Design review of the part built by this model. Coordinates are the model's own, in mm. Face numbers are marked on the shaded views. A direction names the side the tool comes from. Round coordinates to 2 decimals unless told otherwise and drop trailing zeros. Write each loop counter-clockwise with the first axis right and the second up, starting at its lowest first coordinate (ties: lowest second). Pieces come first, ordered by that corner, then holes. Notation, with made-up numbers: (-7.75, -30) -> (-2.75, -30) arc R16 cw to (-2.75, -25) -> close; hole circle Ø4 at (22, -36.5). An arc over 180 degrees is marked (long way). Write item = value, one per line. Start each with the question number.
Item 1: To check wall thickness, follow L1, parallel to Y at x = 36, z = 84; L2, parallel to X at y = 0, z = 26.5; L3, parallel to Y at x = 9, z = 46. State the ranges of each line that lie inside material, in increasing order.
Item 2: Machinability: for the marked faces 4 and 5, which of the approach directions +Z, -Z, +X, -X, +Y, -Y give a long, thin tool a straight path to every point of the face, cutting with its end or side? Answer none if there is none.
Item 3: For pin 1 Ø4 at (y, z) = (2, 61) entering from +X; pin 2 Ø6 at (x, y) = (14, 2.5) entering from +Z; pin 3 Ø6 at (y, z) = (2, 65) entering from -X, all flat-tipped, find the tip position at first contact; note any pin that passes through.
Item 4: Add section A-A, the plane x = 36. State the section outline as (y, z) points.
Item 5: Add section D-D, the plane x = 22.5. State the section outline as (y, z) points.
Item 6: Add section B-B, the plane y = 0. State the section outline as (x, z) points.
Item 7: Add section C-C, the plane z = 6. State the section outline as (x, y) points, then the cut area to 3 significant figures.
Item 8: Mouldability with a two-part tool opening along Y and no side actions: class the marked faces 1, 2 and 3 as released by +Y, released by -Y, zero draft, split by the parting line, or undercut.
from build123d import *

# Parameters (mm, degrees)
SKETCH_1_W      = 44.4
SKETCH_1_H      = 19.4
EXTRUDE_1_DEPTH = 83
FILLET_6_R      = 5
FILLET_7_R      = 5
FILLET_8_R      = 5
FILLET_9_R      = 5
FILLET_11_R     = 2
EXTRUDE_2_DEPTH = 3
EXTRUDE_START   = 3
SKETCH_3_R      = 1.2
EXTRUDE_3_DEPTH = 3


with BuildPart() as part:
    # 草图1 → 凸台-拉伸1 (new body)
    with BuildSketch(Plane.XY):
        with Locations((11.2, 0.3)):
            Rectangle(SKETCH_1_W, SKETCH_1_H)
        Polygon((-9, 6.2), (-9, -5.6), (-7.2, -5.6), (-7.2, -7.4), (29.6, -7.4), (29.6, -5.6), (31.4, -5.6), (31.4, 6.2), (29.6, 6.2), (29.6, 8), (-7.2, 8), (-7.2, 6.2), align=None, mode=Mode.SUBTRACT)
    extrude(amount=EXTRUDE_1_DEPTH)

    # 圆角6
    fillet_6_edges = [part.edges().sort_by_distance(p)[0] for p in [
        (-11, -9.4, 41.5),
    ]]
    fillet(fillet_6_edges, radius=FILLET_6_R)

    # 圆角7
    fillet_7_edges = [part.edges().sort_by_distance(p)[0] for p in [
        (-11, 10, 41.5),
    ]]
    fillet(fillet_7_edges, radius=FILLET_7_R)

    # 圆角8
    fillet_8_edges = [part.edges().sort_by_distance(p)[0] for p in [
        (33.4, 10, 41.5),
    ]]
    fillet(fillet_8_edges, radius=FILLET_8_R)

    # 圆角9
    fillet_9_edges = [part.edges().sort_by_distance(p)[0] for p in [
        (33.4, -9.4, 41.5),
    ]]
    fillet(fillet_9_edges, radius=FILLET_9_R)

    # 圆角11
    # the kernel refuses this fillet: 2 mm, written as the material it takes off along each edge
    with BuildSketch(Plane(origin=(28.4, -9.4, 0), x_dir=(0, 1, 0), z_dir=(-1, 0, 0)), Plane(origin=(-6, 10, 0), x_dir=(0, -1, 0), z_dir=(1, 0, 0))) as fillet_11_piece_1:
        with BuildLine():
            CenterArc((FILLET_11_R, -FILLET_11_R), FILLET_11_R, 90, 90)
            Line((0, -FILLET_11_R), (0, 0))
            Line((0, 0), (FILLET_11_R, 0))
        make_face()
    extrude(amount=34.4, mode=Mode.SUBTRACT)
    with BuildSketch(Plane(origin=(-6, -4.4, 0), x_dir=(0, -1, 0), z_dir=(1, 0, 0))) as fillet_11_piece_2:
        with BuildLine():
            CenterArc((5 - FILLET_11_R, -FILLET_11_R), FILLET_11_R, 0, 90)
            Line((5, -FILLET_11_R), (5, 0))
            Line((5, 0), (5 - FILLET_11_R, 0))
        make_face()
    revolve(axis=Axis((-6, -4.4, 0), (0, 0, -1)), revolution_arc=90, mode=Mode.SUBTRACT)
    with BuildSketch(Plane(origin=(-11, -4.4, 0), x_dir=(1, 0, 0), z_dir=(0, 1, 0)), Plane(origin=(33.4, 5, 0), x_dir=(-1, 0, 0), z_dir=(0, -1, 0))) as fillet_11_piece_3:
        with BuildLine():
            CenterArc((FILLET_11_R, -FILLET_11_R), FILLET_11_R, 90, 90)
            Line((0, -FILLET_11_R), (0, 0))
            Line((0, 0), (FILLET_11_R, 0))
        make_face()
    extrude(amount=9.4, mode=Mode.SUBTRACT)
    with BuildSketch(Plane(origin=(-6, 5, 0), x_dir=(-1, 0, 0), z_dir=(0, -1, 0))) as fillet_11_piece_4:
        with BuildLine():
            CenterArc((5 - FILLET_11_R, -FILLET_11_R), FILLET_11_R, 0, 90)
            Line((5, -FILLET_11_R), (5, 0))
            Line((5, 0), (5 - FILLET_11_R, 0))
        make_face()
    revolve(axis=Axis((-6, 5, 0), (0, 0, -1)), revolution_arc=90, mode=Mode.SUBTRACT)
    with BuildSketch(Plane(origin=(28.4, 5, 0), x_dir=(0, 1, 0), z_dir=(-1, 0, 0))) as fillet_11_piece_5:
        with BuildLine():
            CenterArc((5 - FILLET_11_R, -FILLET_11_R), FILLET_11_R, 0, 90)
            Line((5, -FILLET_11_R), (5, 0))
            Line((5, 0), (5 - FILLET_11_R, 0))
        make_face()
    revolve(axis=Axis((28.4, 5, 0), (0, 0, -1)), revolution_arc=90, mode=Mode.SUBTRACT)
    with BuildSketch(Plane(origin=(28.4, -4.4, 0), x_dir=(1, 0, 0), z_dir=(0, 1, 0))) as fillet_11_piece_6:
        with BuildLine():
            CenterArc((5 - FILLET_11_R, -FILLET_11_R), FILLET_11_R, 0, 90)
            Line((5, -FILLET_11_R), (5, 0))
            Line((5, 0), (5 - FILLET_11_R, 0))
        make_face()
    revolve(axis=Axis((28.4, -4.4, 0), (0, 0, -1)), revolution_arc=90, mode=Mode.SUBTRACT)

    # 草图2 → 凸台-拉伸2 (add)
    with BuildSketch(Plane(origin=(0, 0, 0), x_dir=(-1, 0, 0), z_dir=(0, 0, -1))):
        Polygon((-31.4, 6.2), (-31.4, -5.6), (-29.6, -5.6), (-29.6, -7.4), (7.2, -7.4), (7.2, -5.6), (9, -5.6), (9, 6.2), (7.2, 6.2), (7.2, 8), (-29.6, 8), (-29.6, 6.2), align=None)
    extrude(amount=-EXTRUDE_2_DEPTH)

    # 草图3 → 凸台-拉伸3 (add)
    # profile 1 of 3: a face of its own
    with BuildSketch(Plane.XY.offset(83).offset(EXTRUDE_START)):
        with BuildLine():
            Line((-6, 10), (-16, 10))
            Line((-16, 10), (-16, -9.4))
            Line((-16, -9.4), (-6, -9.4))
            ThreePointArc((-6, -9.4), (-9.535533906, -7.935533906), (-11, -4.4))
            Line((-11, -4.4), (-11, 5))
            ThreePointArc((-11, 5), (-9.535533906, 8.535533906), (-6, 10))
        make_face()
        with Locations((-13.6, -7)):
            Circle(SKETCH_3_R, mode=Mode.SUBTRACT)
        with Locations((-13.6, 7.6)):
            Circle(SKETCH_3_R, mode=Mode.SUBTRACT)
    # profile 2 of 3: a face of its own
    with BuildSketch(Plane.XY.offset(83).offset(EXTRUDE_START)):
        with BuildLine():
            Line((38.4, 10), (28.4, 10))
            ThreePointArc((28.4, 10), (31.935533906, 8.535533906), (33.4, 5))
            Line((33.4, 5), (33.4, -4.4))
            ThreePointArc((33.4, -4.4), (31.935533906, -7.935533906), (28.4, -9.4))
            Line((28.4, -9.4), (38.4, -9.4))
            Line((38.4, -9.4), (38.4, 10))
        make_face()
        with Locations((36, -7)):
            Circle(SKETCH_3_R, mode=Mode.SUBTRACT)
        with Locations((36, 7.6)):
            Circle(SKETCH_3_R, mode=Mode.SUBTRACT)
    # profile 3 of 3: a face of its own
    with BuildSketch(Plane.XY.offset(83).offset(EXTRUDE_START)):
        with BuildLine():
            ThreePointArc((-11, -4.4), (-9.535533906, -7.935533906), (-6, -9.4))
            Line((-6, -9.4), (28.4, -9.4))
            ThreePointArc((28.4, -9.4), (31.935533906, -7.935533906), (33.4, -4.4))
            Line((33.4, -4.4), (33.4, 5))
            ThreePointArc((33.4, 5), (31.935533906, 8.535533906), (28.4, 10))
            Line((28.4, 10), (-6, 10))
            ThreePointArc((-6, 10), (-9.535533906, 8.535533906), (-11, 5))
            Line((-11, 5), (-11, -4.4))
        make_face()
        Polygon((-7.2, -5.6), (-9, -5.6), (-9, 6.2), (-7.2, 6.2), (-7.2, 8), (29.6, 8), (29.6, 6.2), (31.4, 6.2), (31.4, -5.6), (29.6, -5.6), (29.6, -7.4), (-7.2, -7.4), align=None, mode=Mode.SUBTRACT)
    extrude(amount=-EXTRUDE_3_DEPTH)


solid = part.part
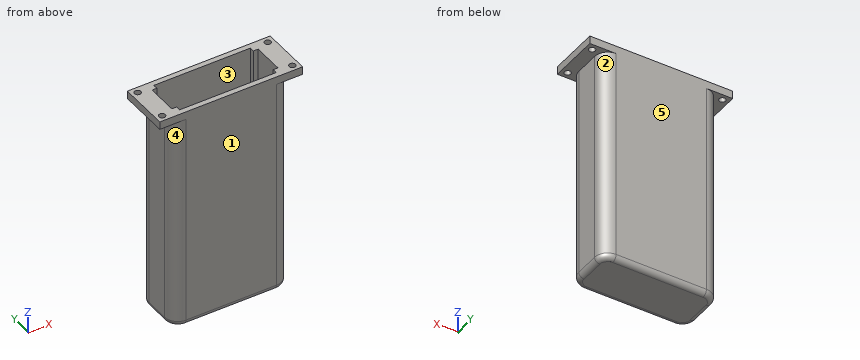
Result set:
q1.L1 = -9.4 to -8.2, -5.8 to 6.4, 8.8 to 10
q1.L2 = -11 to -9, 31.4 to 33.4
q1.L3 = -9.4 to -7.4, 8 to 10
q2.face_4 = -Z, -X, -Y
q2.face_5 = +Z, -Z, +X, -X, +Y
q3.pin_1 = 33.4
q3.pin_2 = 3
q3.pin_3 = -11
q4.outline = (-9.4, 83) -> (-8.2, 83) -> (-8.2, 86) -> (-9.4, 86) -> close; (-5.8, 83) -> (6.4, 83) -> (6.4, 86) -> (-5.8, 86) -> close; (8.8, 83) -> (10, 83) -> (10, 86) -> (8.8, 86) -> close
q5.outline = (-9.4, 2) arc R2 ccw to (-7.4, 0) -> (8, 0) arc R2 ccw to (10, 2) -> (10, 86) -> (8, 86) -> (8, 3) -> (-7.4, 3) -> (-7.4, 86) -> (-9.4, 86) -> close
q6.outline = (-16, 83) -> (-11, 83) -> (-11, 2) arc R2 ccw to (-9, 0) -> (31.4, 0) arc R2 ccw to (33.4, 2) -> (33.4, 83) -> (38.4, 83) -> (38.4, 86) -> (31.4, 86) -> (31.4, 3) -> (-9, 3) -> (-9, 86) -> (-16, 86) -> close
q7.outline = (-11, -4.4) arc R5 ccw to (-6, -9.4) -> (28.4, -9.4) arc R5 ccw to (33.4, -4.4) -> (33.4, 5) arc R5 ccw to (28.4, 10) -> (-6, 10) arc R5 ccw to (-11, 5) -> close; hole (-9, -5.6) -> (-7.2, -5.6) -> (-7.2, -7.4) -> (29.6, -7.4) -> (29.6, -5.6) -> (31.4, -5.6) -> (31.4, 6.2) -> (29.6, 6.2) -> (29.6, 8) -> (-7.2, 8) -> (-7.2, 6.2) -> (-9, 6.2) -> close
q7.area = 231 mm²
q8.face_1 = released by -Y
q8.face_2 = released by +Y
q8.face_3 = undercut
